Here's the drawing with two shaded views (mm, measured from the low corner). I have some questions. Give positions to 0.01 mm unless a question says otherwise; leave off trailing zeros. Loops run counter-clockwise (first coordinate to the right, second up) from the corner with the lowest first, then second, coordinate; pieces in that order, holes last. Notation, with made-up numbers: (11, 49) -> (59, 49) arc R13 ccw to (59, 72) -> close; hole circle Ø4 at (30.5, 51). An arc over 180 degrees is marked (long way). Write each question's results on one line, items separated by ' | '. Start each with the question number.
Q1. If we section it at C-C, the plane z = 0.75: List the corners of the cut face in (x, y) for me.
Q2. If we section it at A-A, the plane x = 15: List the corners of the cut face in (y, z) for me, plus the area to 3 significant figures.
Q3. We'd pull the mould along Y, two halves only. Please class the marked faces 1, 2, 3 and 4: released by +Y, released by -Y, zero draft, split by the parting line, or undercut.
Q4. Will these pins go through, and if not, where does the flat tip stop? P1, Ø3, axis at x = 15, y = 15, coming from the -Z side; P2, Ø3, axis at y = 22.5, z = 2, coming from the -X side; P3, Ø1.1, axis at x = 14.5, y = 15.5, coming from the +Z side.
Q5. If I drill on line 1 along Y through (x, z) = (15, 1.05); line 2 along Z through (x, y) = (7.25, 12); line 3 along Y through (x, z) = (17.75, 3.2), over which ranges is the centre line in solid material (lowest first)?
Q6. If we section it at D-D, the plane z = 4.55: List the corners of the cut face in (x, y) for me, plus the area to 3 significant figures.
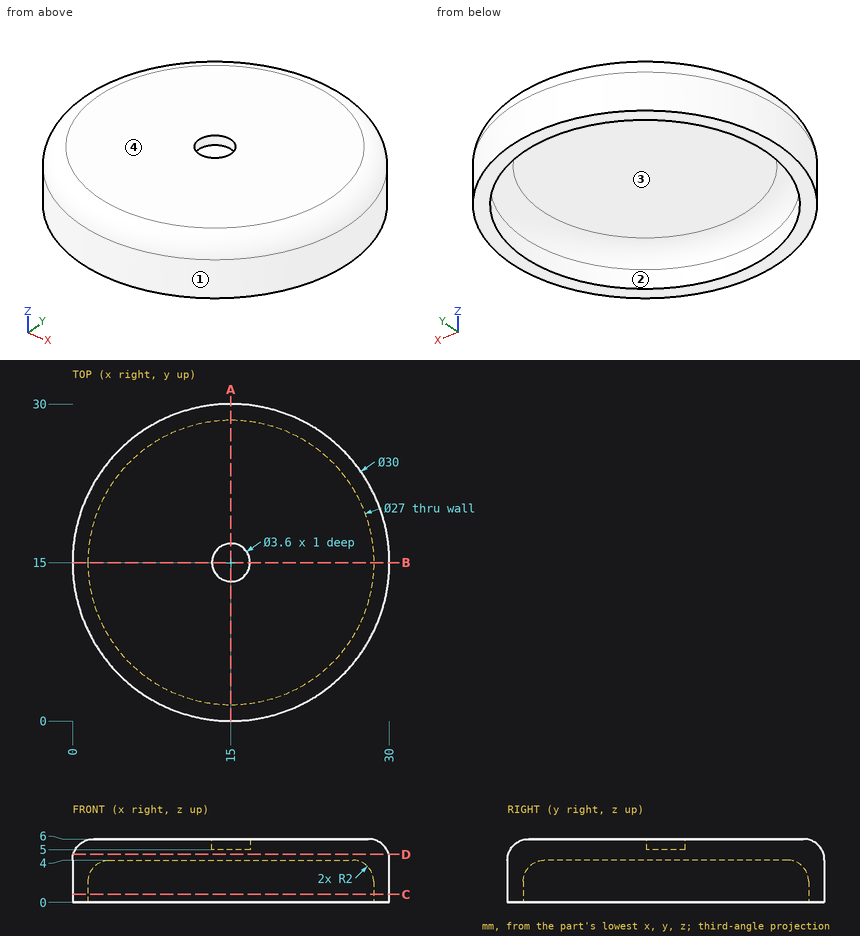
Final values:
1) outline: circle Ø30 at (15, 15); hole circle Ø27 at (15, 15)
2) outline: (0, 0) -> (1.5, 0) -> (1.5, 2) arc R2 cw to (3.5, 4) -> (26.5, 4) arc R2 cw to (28.5, 2) -> (28.5, 0) -> (30, 0) -> (30, 4) arc R2 ccw to (28, 6) -> (16.8, 6) -> (16.8, 5) -> (13.2, 5) -> (13.2, 6) -> (2, 6) arc R2 ccw to (0, 4) -> close | area: 68.4 mm²
3) face 1: split by the parting line | face 2: undercut | face 3: undercut | face 4: zero draft
4) P1: stops at z = 4 | P2: stops at x = 1.25 | P3: stops at z = 5
5) line 1: y = 0 to 1.5, 28.5 to 30 | line 2: z = 4 to 6 | line 3: y = 0.25 to 2.19, 27.81 to 29.75
6) outline: circle Ø29.85 at (15, 15) | area: 700 mm²
